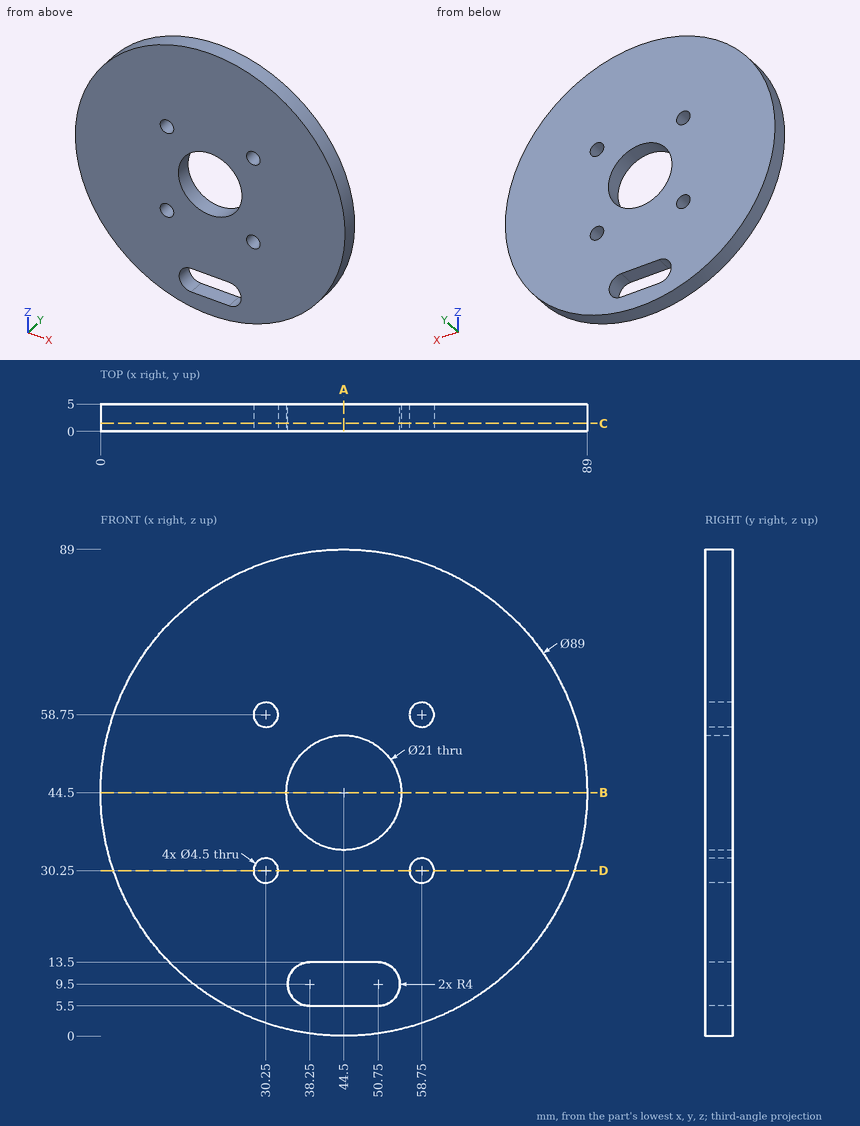
Job drawing, mm, ordinate dimensions from the low corner. One solid piece. Give positions to 0.01 mm unless a question says otherwise; leave off trailing zeros. Loops run counter-clockwise (first coordinate to the right, second up) from the corner with the lowest first, then second, coordinate; pieces in that order, holes last. Notation, with made-up numbers: M 39,70.5 L 87,70.5 A27 cw 87,93.5 Z; hole C 25,88.5 d2. An arc over 180 degrees is marked long. Use one line per item in the form item = value.
Item 1: Drill centre lines: L1, parallel to X at y = 3.55, z = 58; L2, parallel to X at y = 3.6, z = 58.75; L3, parallel to Z at x = 47, y = 1.9. Where is each one in solid material? Low to high.
Filled in:
L1 = 2.1 to 28.13, 32.37 to 56.63, 60.87 to 86.9
L2 = 2.34 to 28, 32.5 to 56.5, 61 to 86.66
L3 = 0.07 to 5.5, 13.5 to 34.3, 54.7 to 88.93
Item 2: Slice it at B-B on z = 44.5. List the corners of the cut face in (x, y), and give its area (3 significant figures).
Filled in:
outline = M 0,0 L 34,0 L 34,5 L 0,5 Z; M 55,0 L 89,0 L 89,5 L 55,5 Z
area = 340 mm^2
Item 3: Flat gauge pins, fed straight in: pin 1 Ø1 at (x, y) = (34, 2) entering from -Z; pin 2 Ø1.5 at (y, z) = (4, 30) entering from -X; pin 3 Ø1.5 at (x, y) = (37, 2) entering from +Z. Where does each tip first touch, or does it go through?
Filled in:
pin_1 = 1.14
pin_2 = 2.18
pin_3 = 88.49
Item 4: Slice it at A-A on x = 44.5. List the corners of the cut face in (y, z), and give its area (3 significant figures).
Filled in:
outline = M 0,0 L 5,0 L 5,5.5 L 0,5.5 Z; M 0,13.5 L 5,13.5 L 5,34 L 0,34 Z; M 0,55 L 5,55 L 5,89 L 0,89 Z
area = 300 mm^2
Item 5: Slice it at C-C on y = 1.45. List the corners of the cut face in (x, z).
Filled in:
outline = C 44.5,44.5 d89; hole C 30.25,30.25 d4.5; hole C 30.25,58.75 d4.5; hole C 44.5,44.5 d21; hole M 38.25,5.5 L 50.75,5.5 A4 ccw 50.75,13.5 L 38.25,13.5 A4 ccw Z; hole C 58.75,30.25 d4.5; hole C 58.75,58.75 d4.5
Item 6: Slice it at D-D on z = 30.25. List the corners of the cut face in (x, y), and give its area (3 significant figures).
Filled in:
outline = M 2.34,0 L 28,0 L 28,5 L 2.34,5 Z; M 32.5,0 L 56.5,0 L 56.5,5 L 32.5,5 Z; M 61,0 L 86.66,0 L 86.66,5 L 61,5 Z
area = 377 mm^2
